The figure shows three views and two pictorial views of one solid part (mm, origin at its lowest corner). Answer the questions. A direction names the side the tool comes from. Coordinates: 2 decimals unless noted, no trailing zeros. Loops run counter-clockwise (first coordinate to the right, second up) from the corner with the lowest first, then second, coordinate; pieces in that order, holes last. Notation, with made-up numbers: M 11.5,24 L 45.5,24 A6 cw 45.5,32 Z; hole C 11,72.5 d8. An arc over 180 degrees is marked long. Write each question's results on one line, items separated by ' | '.
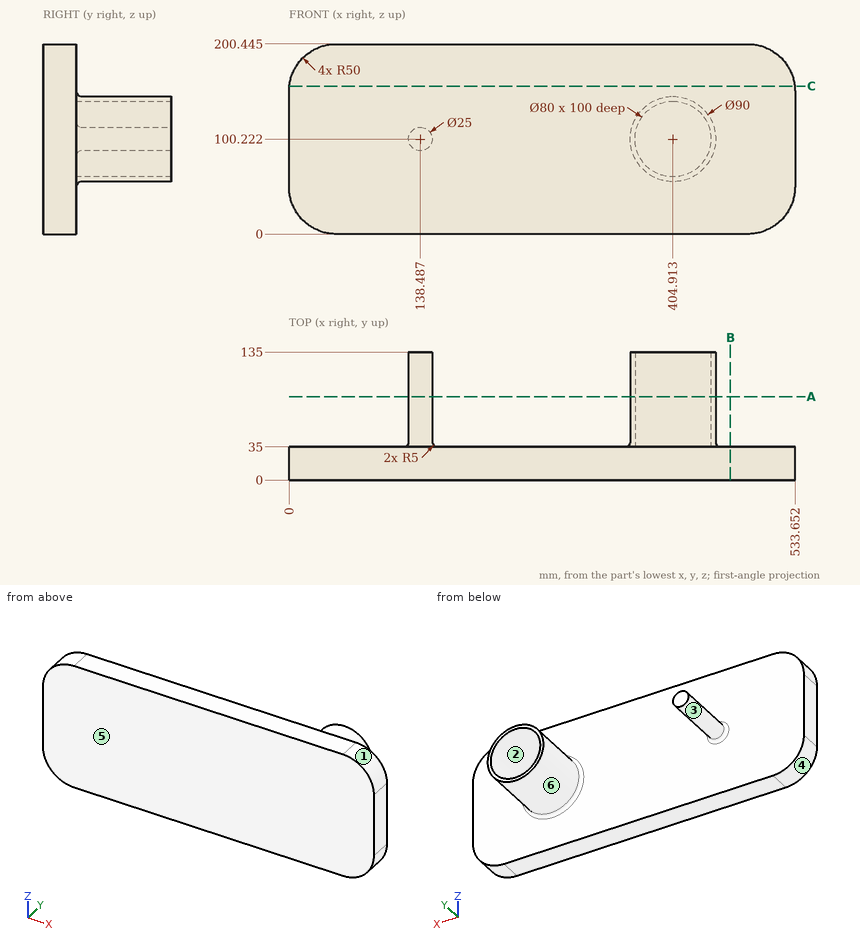
1) Which of the six approach directions +Z, -Z, +X, -X, +Y, -Y give full straight-line access (tool end or side, diameter ignored) to the marked faces 5 and 6?
Check result:
face 5: +Z, -Z, +X, -X, -Y | face 6: +Y
2) For a pull along Z with two mould halves and no side action, classify the marked faces 1, 2, 3 and 4 as released by +Z, released by -Z, zero draft, split by the parting line, or undercut.
Check result:
face 1: released by +Z | face 2: undercut | face 3: split by the parting line | face 4: released by -Z
3) Find section C-C, the plane z = 156. Give the vertices of the cut face in (x, y), and give its area (3 significant figures).
Check result:
outline: M 0.31,0 L 533.34,0 L 533.34,35 L 0.31,35 Z | area: 18,700 mm^2
4) Straight lines are drawn through the part: probe 1 along Y at (x, z) = (302.5, 179.5); probe 2 along X at (y, z) = (99, 80) (1 decimal); probe 3 along X at (y, z) = (86.5, 125.5) (1 decimal). For each, find the intervals that lie inside material, in ascending order. Write a range as [from, to].
Check result:
probe 1: [0, 35] | probe 2: [364.7, 370.4], [439.4, 445.1] | probe 3: [367.7, 373.9], [435.9, 442.1]
5) Find section B-B, the plane x = 465.5. Give the vertices of the cut face in (y, z) (1 decimal), and give its area (3 significant figures).
Check result:
outline: M 0,0 L 35,0 L 35,200.4 L 0,200.4 Z | area: 7,020 mm^2
6) Find section A-A, the plane y = 88. Give the vertices of the cut face in (x, z).
Check result:
outline: C 138.49,100.22 d25; C 404.91,100.22 d90; hole C 404.91,100.22 d80
7) Given pin 1 Ø2 at (x, y) = (144, 40) entering from -Z (1 decimal); pin 2 Ø6 at (y, z) = (62.5, 105) entering from +X; pin 3 Ø12 at (x, y) = (413, 46) entering from +Z, each flat-ended and moving along its own axis, determine where each tip first touches the part or whether it passes through.
Check result:
pin 1: z = 88.6 | pin 2: x = 449.88 | pin 3: z = 145.17
